from build123d import *

# Parameters (mm, degrees)
F0_R     = 62.700464
F2_DEPTH = 25.4
F1_W     = 47.8006
F1_H     = 44.089228
F3_DEPTH = 30
F4_R     = 10


with BuildPart() as f2:
    # F0 (on Front) → F2 (new body)
    with BuildSketch(Plane.XZ):
        Circle(F0_R)
    extrude(amount=F2_DEPTH)

    # F1 (on Front) → F3 (cut)
    with BuildSketch(Plane.XZ):
        Rectangle(F1_W, F1_H)
    extrude(amount=F3_DEPTH, mode=Mode.SUBTRACT)

    # F4
    f4_edges = [f2.edges().sort_by_distance(p)[0] for p in [
        (-62.700464, -25.4, 0),
    ]]
    fillet(f4_edges, radius=F4_R)


solid = f2.part
Geometry: final body of the model. Coordinates: model frame, mm. A direction names the side the tool comes from. Give positions to 0.01 mm unless a question says otherwise; leave off trailing zeros. Loops run counter-clockwise (first coordinate to the right, second up) from the corner with the lowest first, then second, coordinate; pieces in that order, holes last. Notation, with made-up numbers: M 13.5,-36.75 L 39.5,-36.75 A4 cw 39.5,-29.75 Z; hole C 59,-15.5 d3. An arc over 180 degrees is marked long. Put each result on its own line as item: value.
1) Cut plane A-A, the plane z = 0. Return the cut outline in (x, y).
Computed values:
outline: M -62.7,-15.4 A10 ccw -52.7,-25.4 L -23.9,-25.4 L -23.9,0 L -62.7,0 Z; M 23.9,-25.4 L 52.7,-25.4 A10 ccw 62.7,-15.4 L 62.7,0 L 23.9,0 Z
2) First-contact query: P1, Ø6, axis at y = -9, z = -38.5, coming from the -X side; P2, Ø4, axis at x = 25.5, y = -10.5, coming from the +Z side; P3, Ø3, axis at x = 34, y = -23, coming from the +Z side. Flat tips, straight axial feed; report the tip coordinate or a pass-through.
Computed values:
P1: stops at x = -51.68
P2: stops at z = 58.13
P3: stops at z = 50.51
3) Mould query, pull axis Z, two halves, no side actions, for faces 3 (the flat face through (0, -13, 22.045)), 4 (the cylindrical face through (59.805, -7.592, 18.834)), 5 (the flat face through (-1, -25.4, -23)). Classes: released by +Z, released by -Z, zero draft, split by the parting line, or undercut.
Computed values:
face 3: undercut
face 4: split by the parting line
face 5: zero draft
4) Material intervals for L1, parallel to X at y = -3, z = 1.5; L2, parallel to Z at x = 12.5, y = -6.75; L3, parallel to Z at x = 21.5, y = -19, sorted ascending. Write a range as from..to.
Computed values:
L1: x = -62.68..-23.9, 23.9..62.68
L2: z = -61.44..-22.04, 22.04..61.44
L3: z = -58.18..-22.04, 22.04..58.18
5) Reachability of faces 1 (the flat face through (23.9, -13, 0)), 2 (the flat face through (27, 0, 1)) from +Z, -Z, +X, -X, +Y, -Y: full face, straight path, thin tool, end or side. Return the list, or none.
Computed values:
face 1: +Y, -Y
face 2: +Z, -Z, +X, -X, +Y
6) Cut plane C-C, the plane y = -7. Return the cut outline in (x, z).
Computed values:
outline: C 0,0 d125.4; hole M -23.9,-22.04 L 23.9,-22.04 L 23.9,22.04 L -23.9,22.04 Z
7) Cut plane B-B, the plane x = 0. Return the cut outline in (y, z), plus the area to 3 significant figures.
Computed values:
outline: M -25.4,-52.7 A10 ccw -15.4,-62.7 L 0,-62.7 L 0,-22.04 L -25.4,-22.04 Z; M -25.4,22.04 L 0,22.04 L 0,62.7 L -15.4,62.7 A10 ccw -25.4,52.7 Z
area: 2,020 mm^2
